Geometry check sheet. Reference: the model listing, model coordinates, mm. Face numbers are marked on the shaded views. A direction names the side the tool comes from. Coordinates: 2 decimals unless noted, no trailing zeros. Loops run counter-clockwise (first coordinate to the right, second up) from the corner with the lowest first, then second, coordinate; pieces in that order, holes last.
from build123d import *

# Parameters (mm, degrees)
F0_W     = 76.2
F0_H     = 152.4
F1_DEPTH = 12.7
F2_R     = 12.7
F3_DEPTH = 12.7
F4_W     = 25.4
F4_H     = 63.5
F6_W     = 17.78
F6_H     = 15.24
F8_R     = 5.08
F9_SIZE  = 5.08


with BuildPart() as f1:
    # F0 (on Top) → F1 (new body)
    with BuildSketch(Plane.XY):
        Rectangle(F0_W, F0_H)
    extrude(amount=F1_DEPTH)

    # F2 (on Top) → F3 (cut, through all)
    with BuildSketch(Plane.XY):
        with Locations((-17.78, 50.8)):
            Circle(F2_R)
        with Locations((17.78, 50.8)):
            Circle(F2_R)
        with Locations((-17.78, -50.8)):
            Circle(F2_R)
        with Locations((17.78, -50.8)):
            Circle(F2_R)
    extrude(amount=F3_DEPTH, mode=Mode.SUBTRACT)

    # F4 (on Right) → F5 (revolve)
    with BuildSketch(Plane.YZ):
        with Locations((12.7, -31.75)):
            Rectangle(F4_W, F4_H)
    revolve(axis=Axis((0, 0, -31.75), (0, 0, 1)))

    # F6 (on Right) → F7 (revolve, cut)
    with BuildSketch(Plane.YZ):
        with Locations((21.713463, -32.855657)):
            Rectangle(F6_W, F6_H)
    revolve(axis=Axis((0, 0, -63.5), (0, 0, 1)), mode=Mode.SUBTRACT)

    # F8
    f8_edges = [f1.edges().sort_by_distance(p)[0] for p in [
        (0, -25.4, -63.5),
        (0, -25.4, 0),
    ]]
    fillet(f8_edges, radius=F8_R)

    # F9
    f9_edges = [f1.edges().sort_by_distance(p)[0] for p in [
        (-38.1, 0, 0),
        (0, -76.2, 0),
        (38.1, 0, 0),
    ]]
    chamfer(f9_edges, length=F9_SIZE)


solid = f1.part
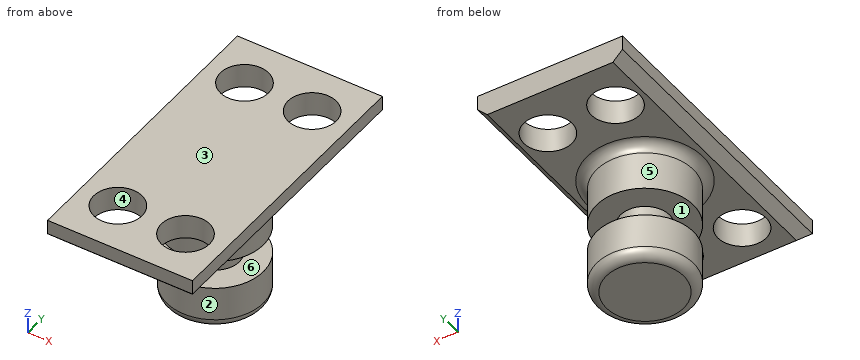
1) Material ranges on probe 1 along Y at (x, z) = (17.78, 7.5); probe 2 along X at (y, z) = (50, 4); probe 3 along Y at (x, z) = (17, 3), recorded low to high.
Data:
probe 1: y = -76.2 to -63.5, -38.1 to 38.1, 63.5 to 76.2
probe 2: x = -37.02 to -30.45, -5.11 to 5.11, 30.45 to 37.02
probe 3: y = -74.12 to -63.48, -38.12 to 38.12, 63.48 to 76.2
2) Section check A-A on z = 2. Record the cut outline in (x, y), and give its area (3 significant figures).
Data:
outline: (-35.02, -73.12) - (35.02, -73.12) - (35.02, 76.2) - (-35.02, 76.2) - close; hole circle Ø25.4 at (-17.78, -50.8); hole circle Ø25.4 at (-17.78, 50.8); hole circle Ø25.4 at (17.78, -50.8); hole circle Ø25.4 at (17.78, 50.8)
area: 8,430 mm2
3) Mould release check, pull along Y, two halves, no side actions. Record for the marked faces 4, 5 and 6: +Y half, -Y half, draft (parallel to the pull), parting line (faces both ways), or undercut.
Data:
face 4: undercut
face 5: parting line
face 6: draft
4) Access from +Z, -Z, +X, -X, +Y, -Y to the whole of each face (thin tool, end or side, straight path). Record for the marked faces 1, 2 and 3.
Data:
face 1: none
face 2: -Z
face 3: +Z, +X, -X, +Y, -Y
5) Section check D-D on y = 40. Record the cut outline in (x, z).
Data:
outline: (-38.1, 5.08) - (-33.02, 0) - (-24.46, 0) - (-24.46, 12.7) - (-38.1, 12.7) - close; (-11.1, 0) - (11.1, 0) - (11.1, 12.7) - (-11.1, 12.7) - close; (24.46, 0) - (33.02, 0) - (38.1, 5.08) - (38.1, 12.7) - (24.46, 12.7) - close
6) Section check C-C on y = 0. Record the cut outline in (x, z), and give its area (3 significant figures).
Data:
outline: (-38.1, 5.08) - (-33.02, 0) - (-30.48, 0) arc R5.08 cw to (-25.4, -5.08) - (-25.4, -25.24) - (-12.82, -25.24) - (-12.82, -40.48) - (-25.4, -40.48) - (-25.4, -58.42) arc R5.08 ccw to (-20.32, -63.5) - (20.32, -63.5) arc R5.08 ccw to (25.4, -58.42) - (25.4, -40.48) - (12.82, -40.48) - (12.82, -25.24) - (25.4, -25.24) - (25.4, -5.08) arc R5.08 cw to (30.48, 0) - (33.02, 0) - (38.1, 5.08) - (38.1, 12.7) - (-38.1, 12.7) - close
area: 3,780 mm2
7) Section check B-B on x = 0. Record the cut outline in (y, z), and give its area (3 significant figures).
Data:
outline: (-76.2, 5.08) - (-71.12, 0) - (-30.48, 0) arc R5.08 cw to (-25.4, -5.08) - (-25.4, -25.24) - (-12.82, -25.24) - (-12.82, -40.48) - (-25.4, -40.48) - (-25.4, -58.42) arc R5.08 ccw to (-20.32, -63.5) - (20.32, -63.5) arc R5.08 ccw to (25.4, -58.42) - (25.4, -40.48) - (12.82, -40.48) - (12.82, -25.24) - (25.4, -25.24) - (25.4, -5.08) arc R5.08 cw to (30.48, 0) - (76.2, 0) - (76.2, 12.7) - (-76.2, 12.7) - close
area: 4,770 mm2
8) Depth check by flat-ended pin: pin 1 (20.5 mm diameter, centred on x = 17.78, y = -50.8, fed in from +Z); pin 2 (12 mm diameter, centred on y = 22, z = -15.5, fed in from -X); pin 3 (12 mm diameter, centred on x = 19, z = -53, fed in from -Y); pin 4 (2 mm diameter, centred on y = -12.5, z = -12.5, fed in from +X). Enter the tip coordinate at first touch or a pass-through.
Data:
pin 1: passes through
pin 2: stops at x = -19.73
pin 3: stops at y = -21.82
pin 4: stops at x = 22.65
